Verification items for the finished model (mm, model axes). Face numbers are marked on the shaded views. Give positions to 0.01 mm unless a question says otherwise; leave off trailing zeros. Answer in a Markdown table with one row per item.
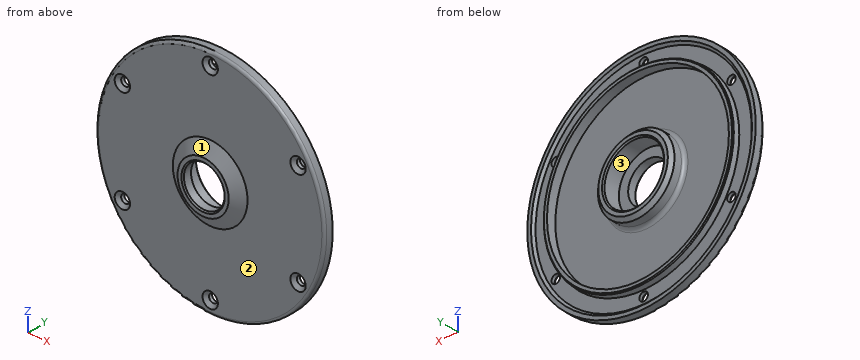
```python
from build123d import *

# Parameters (mm, degrees)
ESQUISSE3_R                               = 2.5
ENL_V_MAT_EXTRU_1_DEPTH                   = 11.85
CHANFREIN1_SIZE                           = 2
R_P_TITION_CIRCULAIRE1_COUNT              = 6
CHANFREIN1_OF_R_P_TITION_CIRCULAIRE1_SIZE = 2


with BuildPart() as part:
    # Esquisse2 → Révolution1 (revolve)
    with BuildSketch(Plane.XY):
        with BuildLine():
            Line((-11.95, 56.6), (-17.45, 56.6))
            Line((-17.45, 56.6), (-17.45, 65.9))
            Line((-17.45, 65.9), (-18.2, 66.65))
            Line((-18.2, 66.65), (-20.4, 66.65))
            Line((-20.4, 66.65), (-22.45, 64.6))
            Line((-22.45, 64.6), (-22.45, 60.1))
            ThreePointArc((-22.45, 60.1), (-23.035786438, 58.685786438), (-24.45, 58.1))
            Line((-24.45, 58.1), (-53.35, 58.1))
            Line((-53.35, 58.1), (-53.35, 63.5))
            Line((-53.35, 63.5), (-55.2, 63.5))
            Line((-55.2, 63.5), (-55.75, 62.95))
            Line((-55.75, 62.95), (-56.1, 59.8))
            Line((-56.1, 59.8), (-63.4, 59.8))
            Line((-63.4, 59.8), (-64.8, 61.2))
            Line((-64.8, 61.2), (-67, 61.2))
            Line((-67, 61.2), (-67, 57.3))
            ThreePointArc((-67, 57.3), (-66.560660172, 56.239339828), (-65.5, 55.8))
            Line((-65.5, 55.8), (-21.9, 55.8))
            Line((-21.9, 55.8), (-15, 51.2))
            Line((-15, 51.2), (-12.7, 51.2))
            Line((-12.7, 51.2), (-11.95, 51.95))
            Line((-11.95, 51.95), (-11.95, 56.6))
        make_face()
    revolve(axis=Axis((0, 0, 0), (0, 1, 0)))

    # Esquisse3 → Enlèv. mat.-Extru.1 (cut, through all)
    with BuildSketch(Plane.XZ.offset(-55.8)):
        with Locations((0, 59.5)):
            Circle(ESQUISSE3_R)
    enl_v_mat_extru_1 = extrude(amount=-ENL_V_MAT_EXTRU_1_DEPTH, mode=Mode.SUBTRACT)

    # Chanfrein1
    chanfrein1_edges = [part.edges().sort_by_distance(p)[0] for p in [
        (-2.5, 55.8, 59.5),
    ]]
    chamfer(chanfrein1_edges, length=CHANFREIN1_SIZE)

    # Répétition circulaire1: Enlèv. mat.-Extru.1 ×6 about axis
    r_p_tition_circulaire1_axis = Axis((0, 0, 0), (0, 1, 0))
    for i in range(1, R_P_TITION_CIRCULAIRE1_COUNT):
        add(enl_v_mat_extru_1.rotate(r_p_tition_circulaire1_axis, i * 360 / R_P_TITION_CIRCULAIRE1_COUNT), mode=Mode.SUBTRACT)

    # Chanfrein1 of Répétition circulaire1
    chanfrein1_of_r_p_tition_circulaire1_edges = [part.edges().sort_by_distance(p)[0] for p in [
        (50.278511525, 55.8, 31.915063509),
        (52.778511525, 55.8, -27.584936491),
        (2.5, 55.8, -59.5),
        (-50.278511525, 55.8, -31.915063509),
        (-52.778511525, 55.8, 27.584936491),
    ]]
    chamfer(chanfrein1_of_r_p_tition_circulaire1_edges, length=CHANFREIN1_OF_R_P_TITION_CIRCULAIRE1_SIZE)


solid = part.part
```
Item 1: Release check for a two-part mould opening along X. For the marked faces 1, 2 and 3 record: released by +X, released by -X, zero draft, split by the parting line, or undercut.
Reported:
| item | result |
|---|---|
| face 1 | split by the parting line |
| face 2 | zero draft |
| face 3 | undercut |
Item 2: Go/stop test with flat-tipped pins: pin 1 (8 mm diameter, centred on x = -50, z = -4.5, fed in from -Y); pin 2 (1.5 mm diameter, centred on y = 60, z = -0.5, fed in from -X); pin 3 (6 mm diameter, centred on x = -51.53, z = 29.75, fed in from -Y); pin 4 (6 mm diameter, centred on x = 51.53, z = 29.75, fed in from +Y). Record where each tip stops, or that it passes through.
Reported:
| item | result |
|---|---|
| pin 1 | stops at y = 55.8 |
| pin 2 | stops at x = -67 |
| pin 3 | stops at y = 57.3 |
| pin 4 | stops at y = 59.8 |
Item 3: Scan lines: L1, parallel to X at y = 61.75, z = 18; L2, parallel to Y at x = 9.5, z = -32; L3, parallel to Z at x = -0.5, y = 59.5. Record each from-to range of solid material in increasing order. Write a range as [from, to].
Reported:
| item | result |
|---|---|
| L1 | x = [-52.91, -50.22], [-13.42, 13.42], [50.22, 52.91] |
| L2 | y = [55.8, 58.1] |
| L3 | z = [-67, -61.95], [-57.05, -53.35], [-22.54, -17.44], [17.44, 22.54], [53.35, 57.05], [61.95, 67] |
Item 4: Sectioned sample at A-A (x = 0). State how many separate pieces and enclosed holes the cut face has, and give its area (3 significant figures).
Reported:
| item | result |
|---|---|
| separate pieces | 4 |
| enclosed holes | 0 |
| area | 403 mm^2 |
